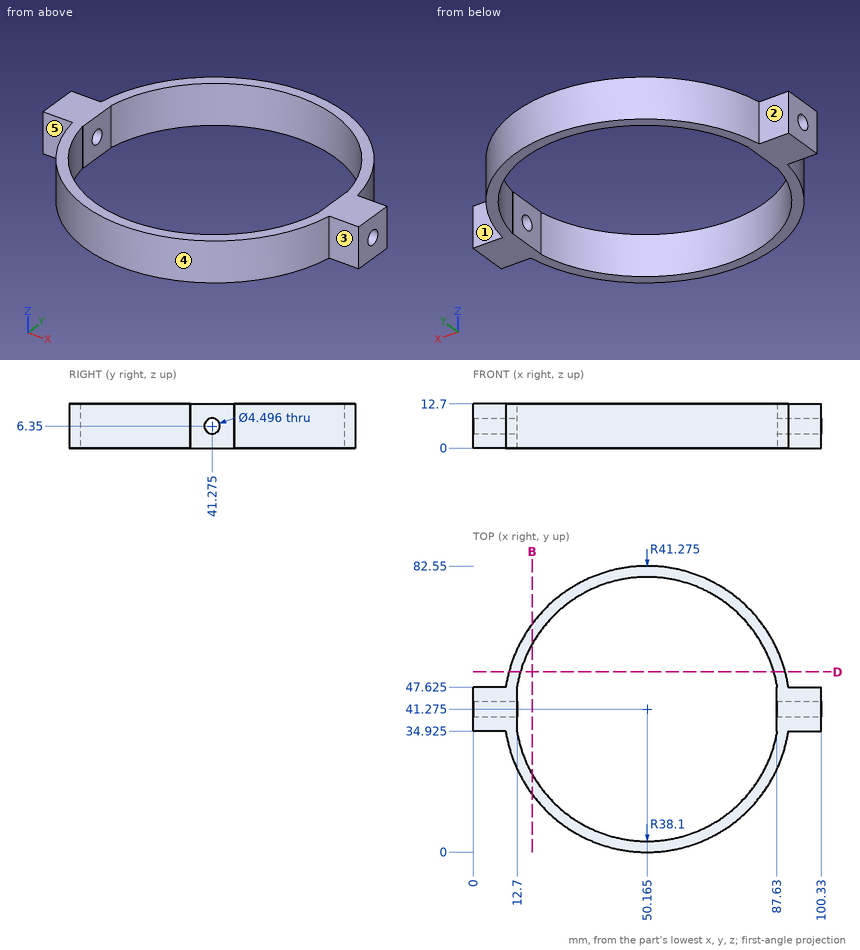
Part print with two shaded views. Sizes in mm from the minimum x, y, z corner. A direction names the side the tool comes from. Coordinates: 2 decimals unless noted, no trailing zeros. Write each loop counter-clockwise with the first axis right and the second up, starting at its lowest first coordinate (ties: lowest second). Pieces come first, ordered by that corner, then holes. Notation, with made-up numbers: (27, 47.25) - (74, 47.25) arc R16 cw to (74, 78.25) - close; hole circle Ø1 at (32.5, 23.5). An arc over 180 degrees is marked (long way). One line per item, written item: value. Start each with the question number.
1. Slice it at D-D (y = 52). Write the cut outline in (x, z).
2. Flat gauge pins, fed straight in: pin 1 (4.5 mm diameter, centred on x = 2.5, z = 9, fed in from +Y) (3 decimals); pin 2 (7 mm diameter, centred on y = 41.275, z = 6.35, fed in from +X); pin 3 (6 mm diameter, centred on x = 18, z = 5.5, fed in from -Y); pin 4 (3 mm diameter, centred on x = 11, y = 61.5, fed in from -Z). Where does each tip first touch, or does it go through?
3. Slice it at B-B (x = 17). Write the cut outline in (y, z).
4. Tool access for the marked faces 1, 2, 3, 4 and 5: list every direction of +Z, -Z, +X, -X, +Y, -Y with a clear straight run to the whole face (end or side of a thin tool).
5. Probe line 1 (X direction, y = 35.5, z = 11.25); line 2 (X direction, y = 67, z = 2.75); line 3 (Y direction, x = 21, z = 7). List the from-to ranges inside material, lowest first. Write a range as from..to.
Answers below:
1. outline: (10.31, 0) - (13.61, 0) - (13.61, 12.7) - (10.31, 12.7) - close; (86.72, 0) - (90.02, 0) - (90.02, 12.7) - (86.72, 12.7) - close
2. pin 1: stops at y = 47.625
2. pin 2: stops at x = 100.33
2. pin 3: stops at y = 12.07
2. pin 4: passes through
3. outline: (16.7, 0) - (22.52, 0) - (22.52, 12.7) - (16.7, 12.7) - close; (60.03, 0) - (65.85, 0) - (65.85, 12.7) - (60.03, 12.7) - close
4. face 1: +Z, -Z, +X, +Y
4. face 2: +Z, -Z, -X, +Y
4. face 3: +Z, -Z, +X, -Y
4. face 4: +Z, -Z, -Y
4. face 5: +Z, -Z, -X, -Y
5. line 1: x = 0..12.7, 87.63..100.33
5. line 2: x = 17.89..22.06, 78.27..82.44
5. line 3: y = 12.07..16.76, 65.79..70.48
